Source: CAD feature listing. Evaluate the final solid. Frame: model axes, mm. A direction names the side the tool comes from. Give positions to 0.01 mm unless a question says otherwise; leave off trailing zeros. Write each loop counter-clockwise with the first axis right and the second up, starting at its lowest first coordinate (ties: lowest second). Pieces come first, ordered by that corner, then holes. Notation, with made-up numbers: (-11, -28) -> (9, -28) arc R4 cw to (9, -23) -> close; hole circle Ø7 at (60.25, 86). An arc over 180 degrees is marked (long way). Use a Markdown table: item, result. Add a question column.
```python
from build123d import *

# Parameters (mm, degrees)
SKETCH_1_W          = 70
SKETCH_1_H          = 20
SKETCH_1_W_2        = 21
SKETCH_1_H_2        = 9
EXTRUDE_1_DEPTH     = 10
CUT_EXTRUDE_1_REACH = 57.98
SKETCH_3_R          = 5.2
SKETCH_3_R_2        = 1
CUT_EXTRUDE_2_REACH = 60.746
SKETCH_4_R          = 1.7


with BuildPart() as part:
    # Sketch 1 → Extrude 1 (new body)
    with BuildSketch(Plane(origin=(0, 0, 0), x_dir=(0.7660444431189771, 0.6427876096865406, 0), z_dir=(-0.6427876096865406, 0.7660444431189771, 0))):
        with Locations((15, 0)):
            Rectangle(SKETCH_1_W, SKETCH_1_H)
        Rectangle(SKETCH_1_W_2, SKETCH_1_H_2, mode=Mode.SUBTRACT)
    extrude(amount=EXTRUDE_1_DEPTH)

    # Sketch 3 → Cut-Extrude 1 (cut, up to next)
    with BuildSketch(Plane(origin=(-6.427876097, 7.660444431, 0), x_dir=(0.7660444431189771, 0.6427876096865406, 0), z_dir=(-0.6427876096865405, 0.766044443118977, 0)), mode=Mode.PRIVATE) as cut_extrude_1_sk1:
        with Locations(Location((39, 0, 0), (0, 0, 180))):
            Circle(SKETCH_3_R)
    cut_extrude_1_tool1 = extrude(cut_extrude_1_sk1.sketch, amount=-CUT_EXTRUDE_1_REACH, mode=Mode.PRIVATE) & part.part
    # Sketch 3 → Cut-Extrude 1 (cut, up to next)
    with BuildSketch(Plane(origin=(-6.427876097, 7.660444431, 0), x_dir=(0.7660444431189771, 0.6427876096865406, 0), z_dir=(-0.6427876096865405, 0.766044443118977, 0)), mode=Mode.PRIVATE) as cut_extrude_1_sk2:
        with Locations(Location((-13, 0, 0), (0, 0, 180))):
            Circle(SKETCH_3_R_2)
    cut_extrude_1_tool2 = extrude(cut_extrude_1_sk2.sketch, amount=-CUT_EXTRUDE_1_REACH, mode=Mode.PRIVATE) & part.part
    # Sketch 3 → Cut-Extrude 1 (cut, up to next)
    with BuildSketch(Plane(origin=(-6.427876097, 7.660444431, 0), x_dir=(0.7660444431189771, 0.6427876096865406, 0), z_dir=(-0.6427876096865405, 0.766044443118977, 0)), mode=Mode.PRIVATE) as cut_extrude_1_sk3:
        with Locations(Location((12, 0, 0), (0, 0, 180))):
            Circle(SKETCH_3_R_2)
    cut_extrude_1_tool3 = extrude(cut_extrude_1_sk3.sketch, amount=-CUT_EXTRUDE_1_REACH, mode=Mode.PRIVATE) & part.part
    add(cut_extrude_1_tool1.solids().sort_by_distance((23.447857, 32.729161, 0))[0], mode=Mode.SUBTRACT)
    add(cut_extrude_1_tool2.solids().sort_by_distance((-16.386454, -0.695794, 0))[0], mode=Mode.SUBTRACT)
    add(cut_extrude_1_tool3.solids().sort_by_distance((2.764657, 15.373896, 0))[0], mode=Mode.SUBTRACT)

    # Sketch 4 → Cut-Extrude 2 (cut, up to next)
    with BuildSketch(Plane.XY.offset(10), mode=Mode.PRIVATE) as cut_extrude_2_sk1:
        with Locations((-16.198218668, -7.064882864)):
            Circle(SKETCH_4_R)
    cut_extrude_2_tool1 = extrude(cut_extrude_2_sk1.sketch, amount=-CUT_EXTRUDE_2_REACH, mode=Mode.PRIVATE) & part.part
    # Sketch 4 → Cut-Extrude 2 (cut, up to next)
    with BuildSketch(Plane.XY.offset(10), mode=Mode.PRIVATE) as cut_extrude_2_sk2:
        with Locations((14.862649296, 18.998279989)):
            Circle(SKETCH_4_R)
    cut_extrude_2_tool2 = extrude(cut_extrude_2_sk2.sketch, amount=-CUT_EXTRUDE_2_REACH, mode=Mode.PRIVATE) & part.part
    add(cut_extrude_2_tool1.solids().sort_by_distance((-16.198219, -7.064883, 10))[0], mode=Mode.SUBTRACT)
    add(cut_extrude_2_tool2.solids().sort_by_distance((14.862649, 18.99828, 10))[0], mode=Mode.SUBTRACT)


solid = part.part
```
(1) Cut plane B-B on z = -6. Return the cut outline in (x, y).
(2) Mould query, pull axis X, two halves, no side actions, for faces 6 (the flat face through (4.7, 17, -0.1)), 7 (the cylindrical face through (-14.58, -6.55, 0.14)), 8 (the flat face through (8, 13, 10)). Classes: +X half, -X half, draft (parallel to the pull), parting line (faces both ways), or undercut.
(3) Cut plane A-A on z = 3.25. Return the cut outline in (x, y).
(4) Access query for faces 1 (the flat face through (-18.49, -9.08, 0.14)), 2 (the flat face through (35.13, 35.92, 0.14)), 3 (the flat face through (-3, 4, 4.5)), 4 (the flat face through (4.87, 10.53, 0.06)), 5 (the flat face through (-11.212, -2.973, 0.063)). Directions: +Z, -Z, +X, -X, +Y, -Y. A direction counts if a zero-diameter tool reaches every point of the face in a straight line with its end or side. Return the directions, or none.
(5) First-contact query: pin 1 Ø4 at (x, y) = (-16.2, -7.06) entering from +Z; pin 2 Ø3 at (x, z) = (12, 3) entering from -Y; pin 3 Ø1.5 at (y, z) = (28, -5) entering from +X; pin 4 Ø2 at (y, z) = (24, -3.5) entering from -X. Flat tips, straight axial feed; report the tip coordinate or a pass-through.
(6) Material intervals for L1, parallel to X at y = 13, z = 0.25; L2, parallel to Y at x = 15, z = -5; L3, parallel to Z at x = -10, y = -8, sorted ascending.
Output:
| question | item | result |
|---|---|---|
| 1 | outline | (-21.75, -5.2) -> (-15.32, -12.86) -> (38.3, 32.14) -> (31.87, 39.8) -> close; hole circle Ø3.4 at (-16.2, -7.06); hole circle Ø3.4 at (14.86, 19) |
| 2 | face 6 | -X half |
| 2 | face 7 | undercut |
| 2 | face 8 | draft |
| 3 | outline | (-21.75, -5.2) -> (-15.32, -12.86) -> (-8.04, -6.75) -> (-14.47, 0.91) -> close; (1.62, 14.41) -> (8.04, 6.75) -> (26.77, 22.46) -> (20.34, 30.12) -> close; (26.56, 35.34) -> (32.99, 27.68) -> (38.3, 32.14) -> (31.87, 39.8) -> close; hole circle Ø3.4 at (-16.2, -7.06); hole circle Ø3.4 at (14.86, 19) |
| 4 | face 1 | +Z, -Z, -X, -Y |
| 4 | face 2 | +Z, -Z, +X, +Y |
| 4 | face 3 | none |
| 4 | face 4 | -X, -Y |
| 4 | face 5 | +X, +Y |
| 5 | pin 1 | z = 10 |
| 5 | pin 2 | y = 8.81 |
| 5 | pin 3 | x = 34.26 |
| 5 | pin 4 | x = 11.85 |
| 6 | L1 | 2.8 to 3.49, 6.02 to 15.49 |
| 6 | L2 | 12.59 to 17.3, 20.69 to 25.64 |
| 6 | L3 | -10 to -0.98, 0.98 to 10 |
